Work out the finished part from the listing and answer in its coordinate system (mm). Face numbers are marked on the shaded views. A direction names the side the tool comes from. Round coordinates to 2 decimals unless told otherwise and drop trailing zeros. Loops run counter-clockwise (first coordinate to the right, second up) from the corner with the lowest first, then second, coordinate; pieces in that order, holes last. Notation, with made-up numbers: (71, 56.5) - (77, 56.5) arc R27 cw to (77, 90.5) - close; hole circle Ø4 at (4, -2). An arc over 180 degrees is marked (long way). Answer as CSV lines item,"result". Start each with the question number.
Q1. Section B-B on z = -84 is taken. Write down the section's boundary in (x, y).
Q2. Section A-A on x = 2 is taken. Write down the section's boundary in (y, z).
Q3. For the marked faces 1 and 2, determine the directions among +Z, -Z, +X, -X, +Y, -Y from which every point of the face is accessible in a straight line to the end or side of a thin tool.
Q4. Section D-D on x = 31 is taken. Write down the section's boundary in (y, z).
Q5. Straight lines are drawn through the part: L1, parallel to Y at x = -8, z = -50; L2, parallel to X at y = -13, z = 106.5. For each, find the intervals that lie inside material, in ascending order. Write a range as [from, to].
Q6. Each of these flat-tipped pins is pushed along its axis until it touches: pin 1 Ø10 at (x, z) = (27, -25.5) entering from -Y; pin 2 Ø6 at (x, z) = (36, 76.5) entering from +Y; pin 3 Ø1.5 at (y, z) = (-15.5, -74.5) entering from +X. Where does it stop, or does it pass through?
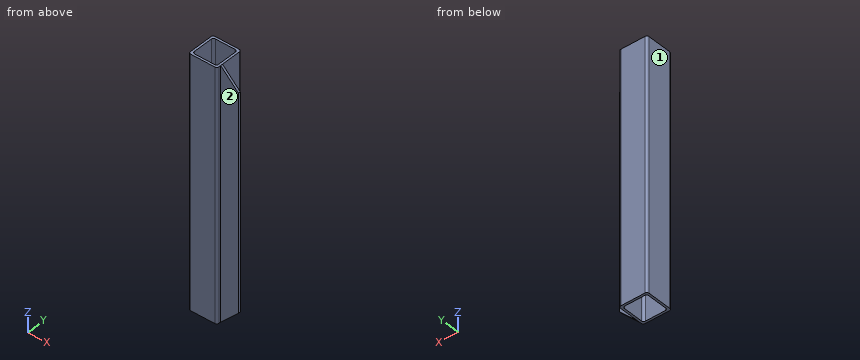
```python
from build123d import *

# Parameters (mm, degrees)
F1_DEPTH = 175
F2_W     = 3
F2_H     = 350
F3_DEPTH = 25
F5_DEPTH = 34.001


# Not quite as in the source:
# - a pattern or mirror of a feature is missing from the dataset's text; its kind, count and spacing are read off the source's solid


with BuildPart() as f1:
    # F0 (on Top) → F1 (new body, symmetric)
    with BuildSketch(Plane.XY):
        with BuildLine():
            ThreePointArc((20, 17), (19.1213203436, 19.1213203436), (17, 20))
            Line((17, 20), (-17, 20))
            ThreePointArc((-17, 20), (-19.1213203436, 19.1213203436), (-20, 17))
            Line((-20, 17), (-20, -17))
            ThreePointArc((-20, -17), (-19.1213203436, -19.1213203436), (-17, -20))
            Line((-17, -20), (17, -20))
            ThreePointArc((17, -20), (19.1213203436, -19.1213203436), (20, -17))
            Line((20, -17), (20, 17))
        make_face()
        with BuildLine():
            ThreePointArc((14, 17), (16.1213203436, 16.1213203436), (17, 14))
            Line((17, 14), (17, -14))
            ThreePointArc((17, -14), (16.1213203436, -16.1213203436), (14, -17))
            Line((14, -17), (-14, -17))
            ThreePointArc((-14, -17), (-16.1213203436, -16.1213203436), (-17, -14))
            Line((-17, -14), (-17, 14))
            ThreePointArc((-17, 14), (-16.1213203436, 16.1213203436), (-14, 17))
            Line((-14, 17), (14, 17))
        make_face(mode=Mode.SUBTRACT)
    extrude(amount=F1_DEPTH, both=True)

    # F2 (on face) → F3 (join)
    with BuildSketch(Plane.YZ.offset(20)):
        with Locations((-12.5, 0)):
            Rectangle(F2_W, F2_H)
    extrude(amount=F3_DEPTH)

    # F4 (on face) → F5 (cut, through all)
    with BuildSketch(Plane.XZ.offset(14)):
        Polygon((45, 175), (20, 175), (45, 150), align=None)
    f5 = extrude(amount=-F5_DEPTH, mode=Mode.SUBTRACT)

    # F5_copies: F5 across plane
    add(f5.mirror(Plane(origin=(0, 0, 0), x_dir=(-1, 0, 0), z_dir=(0, 0, -1))), mode=Mode.SUBTRACT)


solid = f1.part
```
Findings:
1,outline,"(-20, -17) arc R3 ccw to (-17, -20) - (17, -20) arc R3 ccw to (20, -17) - (20, -14) - (45, -14) - (45, -11) - (20, -11) - (20, 17) arc R3 ccw to (17, 20) - (-17, 20) arc R3 ccw to (-20, 17) - close; hole (-17, -14) arc R3 ccw to (-14, -17) - (14, -17) arc R3 ccw to (17, -14) - (17, 14) arc R3 ccw to (14, 17) - (-14, 17) arc R3 ccw to (-17, 14) - close"
2,outline,"(-20, -175) - (-17, -175) - (-17, 175) - (-20, 175) - close; (17, -175) - (20, -175) - (20, 175) - (17, 175) - close"
3,face 1,"+Z, -Z, -X, +Y, -Y"
3,face 2,"+Z, -Z, +X, -Y"
4,outline,"(-14, -164) - (-11, -164) - (-11, 164) - (-14, 164) - close"
5,L1,"y = [-20, -17], [17, 20]"
5,L2,"x = [-20, -17], [17, 45]"
6,pin 1,"stops at y = -14"
6,pin 2,"stops at y = -11"
6,pin 3,"stops at x = 20"
